Build history of the part. All positions in model axes, mm. Face numbers are marked on the shaded views. Coordinates: 2 decimals unless noted, no trailing zeros. Loops run counter-clockwise (first coordinate to the right, second up) from the corner with the lowest first, then second, coordinate; pieces in that order, holes last.
(1) Slice it at C-C (x = 131.5). Give the cut face in (y, z), and give its area (3 significant figures).
(2) Flat gauge pins, fed straight in: P1, Ø1, axis at x = -199.5, z = -243, coming from the +Y side; P2, Ø1, axis at x = 28.5, z = -106, coming from the -Y side; P3, Ø5, axis at x = -162.5, y = -4, coming from the +Z side. Where does each tip first touch, or does it go through?
(3) Slice it at A-A (y = 518.5). Give the cut face in (x, z).
(4) Slice it at B-B (z = -73). Give the cut face in (x, y).
(5) Wall check: L1, parallel to Y at x = -61.5, z = -495; L2, parallel to Y at x = 225, z = -144. Give the ranges that are in metal, low to high.
(6) Slice it at D-D (z = -230). Give the cut face in (x, y), and give its area (3 significant figures).
(7) Two-plate mould, pull along X, no slides. Class the marked faces 1 and 2: pulls with the +X half, pulls with the -X half, needs draft (parallel to the pull), parting line crosses it, or undercut.
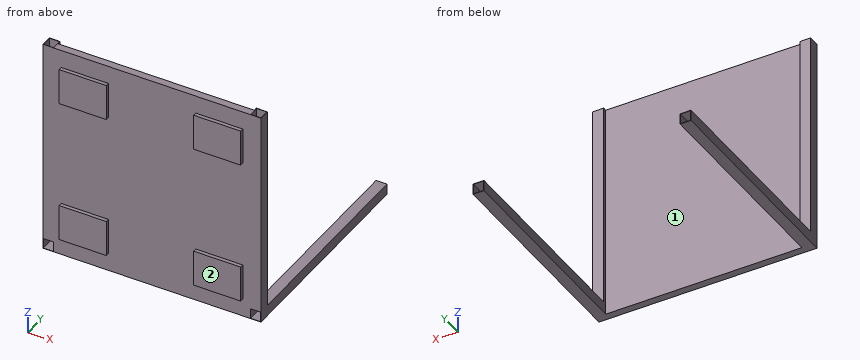
from build123d import *

# Parameters (mm, degrees)
SKETCH1_W                  = 30
SKETCH1_H                  = 30
SKETCH1_W_2                = 28
SKETCH1_H_2                = 28
EXTRUDE_THIN1_DEPTH        = 570
EXTRUDE_THIN1_2_DEPTH      = 570
EXTRUDE_THIN2_DEPTH        = 570
EXTRUDE_THIN2_DEPTH_BACK   = 30
SKETCH3_W                  = 30
SKETCH3_H                  = 30
SKETCH3_W_2                = 28
SKETCH3_H_2                = 28
EXTRUDE_THIN2_2_DEPTH      = 570
EXTRUDE_THIN2_2_DEPTH_BACK = 30
BOSS_EXTRUDE1_DEPTH        = 540
SKETCH5_W                  = 130
SKETCH5_H                  = 100
BOSS_EXTRUDE2_DEPTH        = 10


with BuildPart() as part:
    # Sketch1 → Extrude-Thin1 (new body)
    with BuildSketch(Plane.XY):
        with Locations((-285, 15)):
            Rectangle(SKETCH1_W, SKETCH1_H)
        with Locations((-285, 15)):
            Rectangle(SKETCH1_W_2, SKETCH1_H_2, mode=Mode.SUBTRACT)
    extrude(amount=-EXTRUDE_THIN1_DEPTH)



with BuildPart() as body_2:
    # Sketch1 → Extrude-Thin1 2 (new body)
    with BuildSketch(Plane.XY):
        with Locations((285, 15)):
            Rectangle(SKETCH1_W, SKETCH1_H)
        with Locations((285, 15)):
            Rectangle(SKETCH1_W_2, SKETCH1_H_2, mode=Mode.SUBTRACT)
    extrude(amount=-EXTRUDE_THIN1_2_DEPTH)


with BuildPart() as body_3:
    # Sketch3 → Extrude-Thin2 (new, two sides: drawn at the far end of the back side and taken through both)
    with BuildSketch(Plane(origin=(0, 30, 0), x_dir=(1, 0, 0), z_dir=(0, 1, 0)).offset(-EXTRUDE_THIN2_DEPTH_BACK)):
        with Locations((-285, 585)):
            Rectangle(SKETCH3_W, SKETCH3_H)
        with Locations((-285, 585)):
            Rectangle(SKETCH3_W_2, SKETCH3_H_2, mode=Mode.SUBTRACT)
    extrude(amount=EXTRUDE_THIN2_DEPTH + EXTRUDE_THIN2_DEPTH_BACK)


with BuildPart() as body_4:
    # Sketch3 → Extrude-Thin2 2 (new, two sides: drawn at the far end of the back side and taken through both)
    with BuildSketch(Plane(origin=(0, 30, 0), x_dir=(1, 0, 0), z_dir=(0, 1, 0)).offset(-EXTRUDE_THIN2_2_DEPTH_BACK)):
        with Locations((285, 585)):
            Rectangle(SKETCH3_W, SKETCH3_H)
        with Locations((285, 585)):
            Rectangle(SKETCH3_W_2, SKETCH3_H_2, mode=Mode.SUBTRACT)
    extrude(amount=EXTRUDE_THIN2_2_DEPTH + EXTRUDE_THIN2_2_DEPTH_BACK)


with BuildPart() as part_1:
    add(part.part)

    add(body_2.part)  # Boss-Extrude1 merges body 2

    add(body_3.part)  # Boss-Extrude1 merges body 3

    add(body_4.part)  # Boss-Extrude1 merges body 4
    # Sketch4 → Boss-Extrude1 (add)
    with BuildSketch(Plane(origin=(-270, 0, 0), x_dir=(0, 0, -1), z_dir=(1, 0, 0))):
        Polygon((600, 0), (600, 20), (570, 20), (0, 20), (0, 0), (570, 0), align=None)
    extrude(amount=BOSS_EXTRUDE1_DEPTH)

    # Sketch5 → Boss-Extrude2 (add)
    with BuildSketch(Plane(origin=(0, 0, 0), x_dir=(-1, 0, 0), z_dir=(0, -1, 0))):
        with Locations((-185, 500)):
            Rectangle(SKETCH5_W, SKETCH5_H)
        with Locations((185, 500)):
            Rectangle(SKETCH5_W, SKETCH5_H)
        with Locations((185, 100)):
            Rectangle(SKETCH5_W, SKETCH5_H)
        with Locations((-185, 100)):
            Rectangle(SKETCH5_W, SKETCH5_H)
    extrude(amount=BOSS_EXTRUDE2_DEPTH)


solid = part_1.part
Response values:
1. outline: (-10, -550) - (0, -550) - (0, -600) - (20, -600) - (20, 0) - (0, 0) - (0, -50) - (-10, -50) - (-10, -150) - (0, -150) - (0, -450) - (-10, -450) - close
1. area: 14,000 mm2
2. P1: stops at y = 20
2. P2: stops at y = 0
2. P3: stops at z = -50
3. outline: (-300, -600) - (-270, -600) - (-270, -570) - (-300, -570) - close; (270, -600) - (300, -600) - (300, -570) - (270, -570) - close; hole (-299, -599) - (-271, -599) - (-271, -571) - (-299, -571) - close; hole (271, -599) - (299, -599) - (299, -571) - (271, -571) - close
4. outline: (-300, 0) - (-250, 0) - (-250, -10) - (-120, -10) - (-120, 0) - (120, 0) - (120, -10) - (250, -10) - (250, 0) - (300, 0) - (300, 30) - (270, 30) - (270, 20) - (-270, 20) - (-270, 30) - (-300, 30) - close; hole (-299, 1) - (-271, 1) - (-271, 29) - (-299, 29) - close; hole (271, 1) - (299, 1) - (299, 29) - (271, 29) - close
5. L1: y = 0 to 20
5. L2: y = -10 to 20
6. outline: (-300, 0) - (300, 0) - (300, 30) - (270, 30) - (270, 20) - (-270, 20) - (-270, 30) - (-300, 30) - close; hole (-299, 1) - (-271, 1) - (-271, 29) - (-299, 29) - close; hole (271, 1) - (299, 1) - (299, 29) - (271, 29) - close
6. area: 11,000 mm2
7. face 1: undercut
7. face 2: needs draft
